```python
from build123d import *

# Parameters (mm, degrees)
F0_W     = 200
F0_H     = 100
F1_DEPTH = 7.4
F2_W     = 8
F2_H     = 2.7
F3_DEPTH = 2
F4_W     = 108
F4_H     = 50
F5_DEPTH = 7.401
F6_SCALE = 5


with BuildPart() as f1:
    # F0 (on Front) → F1 (new body)
    with BuildSketch(Plane.XZ):
        with Locations((2.2038258612, 6.3567497451)):
            Rectangle(F0_W, F0_H)
    extrude(amount=F1_DEPTH)

    # F2 (on face) → F3 (join)
    with BuildSketch(Plane.XZ.offset(7.4)):
        with Locations((-93.7961741388, 55.0067497451)):
            Rectangle(F2_W, F2_H)
        with Locations((98.2038258612, 55.0067497451)):
            Rectangle(F2_W, F2_H)
        with Locations((98.2038258612, -42.2932502549)):
            Rectangle(F2_W, F2_H)
        with Locations((-93.7961741388, -42.2932502549)):
            Rectangle(F2_W, F2_H)
    extrude(amount=F3_DEPTH)

    # F4 (on face) → F5 (cut, through all)
    with BuildSketch(Plane.XZ.offset(7.4)):
        Rectangle(F4_W, F4_H)
    extrude(amount=-F5_DEPTH, mode=Mode.SUBTRACT)


with BuildPart() as f1_1:
    # F6: moved
    add(f1.part.scale(F6_SCALE))


solid = f1_1.part
```
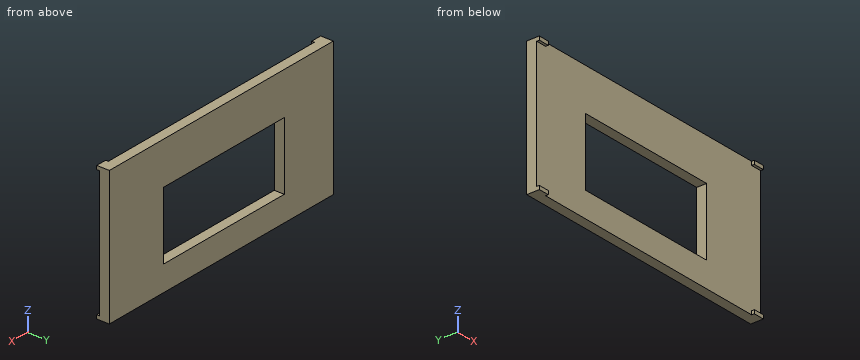
The model under review builds one solid part; all positions refer to its coordinate system, in mm. Round coordinates to 2 decimals unless told otherwise and drop trailing zeros. Loops run counter-clockwise (first coordinate to the right, second up) from the corner with the lowest first, then second, coordinate; pieces in that order, holes last. Notation, with made-up numbers: (43.5, 26.5) - (65.5, 26.5) arc R19 ccw to (65.5, 44.5) - close; hole circle Ø10 at (-29.5, 68). An arc over 180 degrees is marked (long way). Write each question's results on one line, items separated by ' | '. Start each with the question number.
Q1. Take a section at C-C on z = -2. Give the boundary of the cut face in (x, y), plus the area to 3 significant figures.
Q2. Take a section at A-A on x = -120.5. Give the boundary of the cut face in (y, z), plus the area to 3 significant figures.
Q3. Take a section at B-B on y = -28. Give the boundary of the cut face in (x, z), plus the area to 3 significant figures.
Q4. Insertion check: P1, Ø12, axis at x = 134.5, z = -150.5, coming from the -Y side. The pin has a flat end and moves straight along its axis. Give the tip position at first contact, or say it passes through.
Q5. Take a section at D-D on z = 244.5. Give the boundary of the cut face in (x, y).
Q6. Wall thickness on line 1 along X through (y, z) = (-25, 105); line 2 along Z through (x, y) = (-41, -32); line 3 along Y through (x, z) = (104, 162.5): over which ranges is each line inside the solid? List them lowest first. Write a range as [from, to].
Data:
1) outline: (-488.98, -37) - (-270, -37) - (-270, 0) - (-488.98, 0) - close; (270, -37) - (511.02, -37) - (511.02, 0) - (270, 0) - close | area: 17,000 mm²
2) outline: (-37, -218.22) - (0, -218.22) - (0, -125) - (-37, -125) - close; (-37, 125) - (0, 125) - (0, 281.78) - (-37, 281.78) - close | area: 9,250 mm²
3) outline: (-488.98, -218.22) - (511.02, -218.22) - (511.02, 281.78) - (-488.98, 281.78) - close; hole (-270, -125) - (270, -125) - (270, 125) - (-270, 125) - close | area: 365,000 mm²
4) P1: stops at y = -37
5) outline: (-488.98, -37) - (511.02, -37) - (511.02, 0) - (-488.98, 0) - close
6) line 1: x = [-488.98, -270], [270, 511.02] | line 2: z = [-218.22, -125], [125, 281.78] | line 3: y = [-37, 0]
